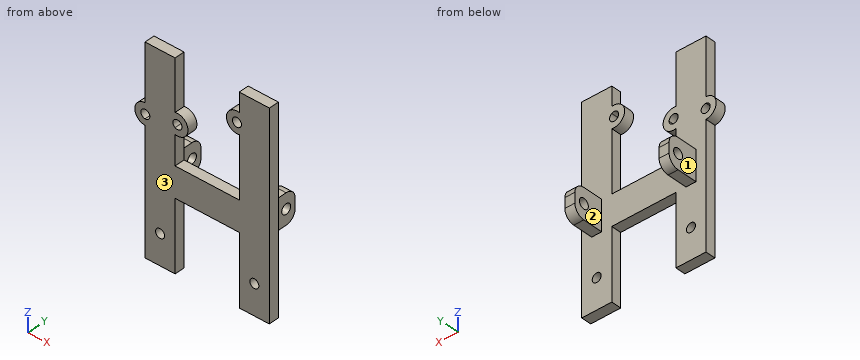
from build123d import *

# Parameters (mm, degrees)
SKETCH1_W           = 15
SKETCH1_H           = 100
SKETCH1_W_2         = 32
SKETCH1_H_2         = 15
BOSS_EXTRUDE1_DEPTH = 2.5
SKETCH2_W           = 5
SKETCH2_H           = 15
BOSS_EXTRUDE2_DEPTH = 15
SKETCH3_R           = 2.5
CUT_EXTRUDE1_DEPTH  = 52
FILLET2_R           = 5
BOSS_EXTRUDE3_DEPTH = 5
SKETCH5_R           = 2.25
CUT_EXTRUDE3_DEPTH  = 5
SKETCH6_R           = 2.25
CUT_EXTRUDE4_DEPTH  = 5


with BuildPart() as part:
    # Sketch1 → Boss-Extrude1 (new body, symmetric)
    with BuildSketch(Plane(origin=(0, 0, 0), x_dir=(1, 0, 0), z_dir=(0, 1, 0))):
        with Locations((7.5, 50)):
            Rectangle(SKETCH1_W, SKETCH1_H)
        with Locations((31, 57.5)):
            Rectangle(SKETCH1_W_2, SKETCH1_H_2)
        with Locations((54.5, 50)):
            Rectangle(SKETCH1_W, SKETCH1_H)
    extrude(amount=BOSS_EXTRUDE1_DEPTH, both=True)

    # Sketch2 → Boss-Extrude2 (add)
    with BuildSketch(Plane(origin=(0, 2.5, 0), x_dir=(1, 0, 0), z_dir=(0, 1, 0))):
        with Locations((54.5, 57.5)):
            Rectangle(SKETCH2_W, SKETCH2_H)
        with Locations((7.5, 57.5)):
            Rectangle(SKETCH2_W, SKETCH2_H)
    extrude(amount=BOSS_EXTRUDE2_DEPTH)

    # Sketch3 → Cut-Extrude1 (cut)
    with BuildSketch(Plane.ZY.offset(-5)):
        with Locations((-57.5, 12.5)):
            Circle(SKETCH3_R)
    extrude(amount=-CUT_EXTRUDE1_DEPTH, mode=Mode.SUBTRACT)

    # Fillet2
    fillet2_edges = [part.edges().sort_by_distance(p)[0] for p in [
        (54.5, 17.5, -65),
        (54.5, 17.5, -50),
        (7.5, 17.5, -65),
        (7.5, 17.5, -50),
    ]]
    fillet(fillet2_edges, radius=FILLET2_R)

    # Sketch4 → Boss-Extrude3 (add)
    with BuildSketch(Plane(origin=(0, 2.5, 0), x_dir=(1, 0, 0), z_dir=(0, 1, 0))):
        with BuildLine():
            ThreePointArc((47, 12.674737063), (43.587769422, 14.601319551), (47, 16.527902039))
            Line((47, 16.527902039), (47, 19.721057834))
            ThreePointArc((47, 19.721057834), (40.587769422, 14.601319551), (47, 9.481581269))
            Line((47, 9.481581269), (47, 12.674737063))
        make_face()
        with BuildLine():
            ThreePointArc((15, 25.231075416), (21.41, 30.351319551), (15, 35.471563686))
            Line((15, 35.471563686), (15, 32.279245898))
            ThreePointArc((15, 32.279245898), (17.26736173, 32.30995428), (18.41, 30.351319551))
            ThreePointArc((18.41, 30.351319551), (17.26736173, 28.392684823), (15, 28.423393204))
            Line((15, 28.423393204), (15, 25.231075416))
        make_face()
        with BuildLine():
            Line((0, 35.595623452), (0, 38.59888089))
            ThreePointArc((0, 38.59888089), (-5.09, 33.351319551), (0, 28.103758213))
            Line((0, 28.103758213), (0, 31.10701565))
            ThreePointArc((0, 31.10701565), (-2.09, 33.351319551), (0, 35.595623452))
        make_face()
    extrude(amount=-BOSS_EXTRUDE3_DEPTH)

    # Sketch5 → Cut-Extrude3 (cut)
    with BuildSketch(Plane(origin=(0, 2.5, 0), x_dir=(1, 0, 0), z_dir=(0, 1, 0))):
        with Locations((0.16, 33.351319551)):
            Circle(SKETCH5_R)
        with Locations((16.16, 30.351319551)):
            Circle(SKETCH5_R)
        with Locations((45.837769422, 14.601319551)):
            Circle(SKETCH5_R)
    extrude(amount=-CUT_EXTRUDE3_DEPTH, mode=Mode.SUBTRACT)

    # Sketch6 → Cut-Extrude4 (cut)
    with BuildSketch(Plane(origin=(0, 2.5, 0), x_dir=(1, 0, 0), z_dir=(0, 1, 0))):
        with Locations((7.5, 85)):
            Circle(SKETCH6_R)
        with Locations((54.5, 85)):
            Circle(SKETCH6_R)
    extrude(amount=-CUT_EXTRUDE4_DEPTH, mode=Mode.SUBTRACT)


solid = part.part
The listing builds one solid part. Answer for the finished solid, in the listing's coordinates (mm). Face numbers are marked on the shaded views. Coordinates: 2 decimals unless noted, no trailing zeros. Loops run counter-clockwise (first coordinate to the right, second up) from the corner with the lowest first, then second, coordinate; pieces in that order, holes last.
1) Flat-ended cylindrical pins translate along their axes: pin 1 Ø12 at (y, z) = (10.5, -56.5) entering from -X; pin 2 Ø2 at (x, y) = (13, 4) entering from +Z; pin 3 Ø8 at (y, z) = (12, -51.5) entering from +X; pin 4 Ø1.5 at (x, y) = (55, 9.5) entering from +Z. Find the tip coordinate at first contact, or state that the pin passes through.
2) Find section B-B on z = -85. Write down the section's boundary in (x, y), then the cut area to 3 significant figures.
3) Find section A-A on x = 7.5. Write down the section's boundary in (y, z).
4) Find section C-C on y = 7.5. Write down the section's boundary in (x, z).
5) Determine the mould class of the marked faces 1, 2 and 3 for opening direction X: pulls with the +X half, pulls with the -X half, needs draft (parallel to the pull), parting line crosses it, or undercut.
6) Find section D-D on y = 1. Write down the section's boundary in (x, z).
7) Find the intervals of material crossed by L1, parallel to X at y = -1.2, z = -85; L2, parallel to X at y = 7, z = -53; L3, parallel to Y at x = 8.7, z = -57.5, in increasing order.
Values:
1. pin 1: stops at x = 5
1. pin 2: passes through
1. pin 3: stops at x = 57
1. pin 4: stops at z = -50
2. outline: (0, -2.5) - (5.25, -2.5) - (5.25, 2.5) - (0, 2.5) - close; (9.75, -2.5) - (15, -2.5) - (15, 2.5) - (9.75, 2.5) - close; (47, -2.5) - (52.25, -2.5) - (52.25, 2.5) - (47, 2.5) - close; (56.75, -2.5) - (62, -2.5) - (62, 2.5) - (56.75, 2.5) - close
2. area: 105 mm2
3. outline: (-2.5, -100) - (2.5, -100) - (2.5, -87.25) - (-2.5, -87.25) - close; (-2.5, -82.75) - (2.5, -82.75) - (2.5, -65) - (12.5, -65) arc R5 ccw to (17.5, -60) - (17.5, -55) arc R5 ccw to (12.5, -50) - (2.5, -50) - (2.5, 0) - (-2.5, 0) - close; hole circle Ø5 at (12.5, -57.5)
4. outline: (5, -65) - (10, -65) - (10, -50) - (5, -50) - close; (52, -65) - (57, -65) - (57, -50) - (52, -50) - close
5. face 1: pulls with the -X half
5. face 2: undercut
5. face 3: needs draft
6. outline: (0, -100) - (15, -100) - (15, -65) - (47, -65) - (47, -100) - (62, -100) - (62, 0) - (47, 0) - (47, -9.48) arc R5.25 ccw (long way) to (47, -19.72) - (47, -50) - (15, -50) - (15, -35.47) arc R5.25 ccw (long way) to (15, -25.23) - (15, 0) - (0, 0) - (0, -28.1) arc R5.25 ccw to (0, -38.6) - close; hole circle Ø4.5 at (0.16, -33.35); hole circle Ø4.5 at (7.5, -85); hole circle Ø4.5 at (16.16, -30.35); hole circle Ø4.5 at (45.84, -14.6); hole circle Ø4.5 at (54.5, -85)
7. L1: x = 0 to 5.25, 9.75 to 15, 47 to 52.25, 56.75 to 62
7. L2: x = 5 to 10, 52 to 57
7. L3: y = -2.5 to 10, 15 to 17.5
